Model file for the job. Use its own axes, mm. Coordinates: 2 decimals unless noted, no trailing zeros. Write each loop counter-clockwise with the first axis right and the second up, starting at its lowest first coordinate (ties: lowest second). Pieces come first, ordered by that corner, then holes. Notation, with made-up numbers: (-25.5, 72.5) - (19.5, 72.5) arc R10 cw to (19.5, 82.5) - close; hole circle Ø11 at (66, 69). An arc over 180 degrees is marked (long way). Put each result on its own line as item: value. Start each with the question number.
1. Saw through at A-A, the plane x = 0. Write the cut outline in (y, z), plus the area to 3 significant figures.
2. Saw through at D-D, the plane z = -11. Write the cut outline in (x, y), plus the area to 3 significant figures.
3. Saw through at B-B, the plane z = 0. Write the cut outline in (x, y), plus the area to 3 significant figures.
4. Drill centre lines: L1, parallel to Z at x = 0, y = 117.5; L2, parallel to X at y = 96, z = 2. Where is each one in solid material? Low to high. Write a range as from..to.
5. Pull direction Z, two halves, no side cores. Call faces 1 (the face through (-22, 200, 0)), 2 (the face through (7.509, 98.6, 23.846)), 3 (the face through (22.39, 192.52, -0.33)), 4 (the face through (1.7, 181, -20.2)): released by +Z, released by -Z, zero draft, split by the parting line, or undercut.
6. Drop flat-ended pins along their axis: P1, Ø4, axis at y = 43, z = -11.5, coming from the +X side; P2, Ø12, axis at x = -6.5, y = 25.5, coming from the +Z side (3 decimals); P3, Ø8, axis at y = 147, z = 6, coming from the +X side. Give the stop position or say it passes through.
7. Saw through at C-C, the plane y = 195. Write the cut outline in (x, z).
```python
from build123d import *

# Parameters (mm, degrees)
SKETCH1_R               = 25
SKETCH1_R_2             = 20
BOSS_EXTRUDE1_DEPTH     = 200
CUT_EXTRUDE1_DEPTH      = 200
CUT_EXTRUDE1_DEPTH_BACK = 200
SKETCH2_R               = 2.5


with BuildPart() as part:
    # Sketch1 → Boss-Extrude1 (new body)
    with BuildSketch(Plane(origin=(0, 0, 0), x_dir=(1, 0, 0), z_dir=(0, 1, 0))):
        with Locations(Location((0, 0, 0), (0, 0, 270))):
            Circle(SKETCH1_R)
        with Locations(Location((0, 0, 0), (0, 0, 270))):
            Circle(SKETCH1_R_2, mode=Mode.SUBTRACT)
    extrude(amount=BOSS_EXTRUDE1_DEPTH)

    # Sketch2 → Cut-Extrude1 (cut, two sides: drawn at the far end of the back side and taken through both)
    with BuildSketch(Plane(origin=(0, 0, 0), x_dir=(0, 0, -1), z_dir=(1, 0, 0)).offset(-CUT_EXTRUDE1_DEPTH_BACK)):
        with Locations(Location((0, 195, 0), (0, 0, 180))):
            Circle(SKETCH2_R)
        Polygon((25, 175), (5, 200), (-5, 200), (-25, 175), (-25, 205.937261936), (25, 205.937261936), align=None)
    extrude(amount=CUT_EXTRUDE1_DEPTH + CUT_EXTRUDE1_DEPTH_BACK, mode=Mode.SUBTRACT)


solid = part.part
```
Final values:
1. outline: (0, -25) - (175, -25) - (181.25, -20) - (0, -20) - close; (0, 20) - (181.25, 20) - (175, 25) - (0, 25) - close
1. area: 1,780 mm²
2. outline: (-22.45, 0) - (-16.7, 0) - (-16.7, 192.5) - (-22.45, 192.5) - close; (16.7, 0) - (22.45, 0) - (22.45, 192.5) - (16.7, 192.5) - close
2. area: 2,210 mm²
3. outline: (-25, 0) - (-20, 0) - (-20, 192.5) - (-25, 192.5) - close; (-25, 197.5) - (-20, 197.5) - (-20, 200) - (-25, 200) - close; (20, 0) - (25, 0) - (25, 192.5) - (20, 192.5) - close; (20, 197.5) - (25, 197.5) - (25, 200) - (20, 200) - close
3. area: 1,950 mm²
4. L1: z = -25..-20, 20..25
4. L2: x = -24.92..-19.9, 19.9..24.92
5. face 1: zero draft
5. face 2: split by the parting line
5. face 3: undercut
5. face 4: released by -Z
6. P1: stops at x = 23.12
6. P2: stops at z = 24.995
6. P3: stops at x = 24.92
7. outline: (-24.87, -2.5) arc R25 ccw to (-23.32, -9) - (-17.86, -9) arc R20 cw to (-19.84, -2.5) - close; (-24.87, 2.5) - (-19.84, 2.5) arc R20 cw to (-17.86, 9) - (-23.32, 9) arc R25 ccw to start; (17.86, -9) - (23.32, -9) arc R25 ccw to (24.87, -2.5) - (19.84, -2.5) arc R20 cw to start; (17.86, 9) arc R20 cw to (19.84, 2.5) - (24.87, 2.5) arc R25 ccw to (23.32, 9) - close
